Read the model definition and answer for the solid it produces. Units are mm, in the model's axes. Face numbers are marked on the shaded views. A direction names the side the tool comes from. Coordinates: 2 decimals unless noted, no trailing zeros. Write each loop counter-clockwise with the first axis right and the second up, starting at its lowest first coordinate (ties: lowest second). Pieces come first, ordered by that corner, then holes.
(1) Find the intervals of material crossed by probe 1 along Y at (x, z) = (38, -181.5); probe 2 along Z at (x, y) = (21, -173); probe 3 along X at (y, z) = (-77, -86.5), in increasing order.
(2) Which of the six approach directions +Z, -Z, +X, -X, +Y, -Y give full straight-line access (tool end or side, diameter ignored) to the marked faces 1 and 2?
(3) Section A-A on x = 16 is taken. Write down the section's boundary in (y, z).
(4) Section C-C on y = -151 is taken. Write down the section's boundary in (x, z).
(5) The mould has two halves that part along Z. Classify the marked faces 3, 4 and 5: +Z half, -Z half, draft (parallel to the pull), parting line (faces both ways), or undercut.
(6) Section B-B on z = -127.5 is taken. Write down the section's boundary in (x, y).
Autodesk Inventor part; units mm, degrees
ref_plane "YZ Plane" through (0, 0, 0) normal (1, 0, 0) x (0, 1, 0)
ref_plane "XZ Plane" through (0, 0, 0) normal (0, 1, 0) x (-1, 0, 0)
ref_plane "XY Plane" through (0, 0, 0) normal (0, 0, 1) x (1, 0, 0)
ref_plane "РабПлоскость1" through (8, 0, 0) normal (1, 0, 0) x (0, 0, -1)
sketch "Эскиз2" plane through (8, 0, 0) normal (1, 0, 0) x (0, 0, -1)
  line L0 (200, 300) -> (-200, 300)
  line L1 (200, -300) -> (200, 300)
  line L2 (-200, 300) -> (200, 300)
  line L3 (200, 300) -> (200, -300)
  line L4 (200, -300) -> (-200, -300)
  line L5 (-200, -300) -> (-200, 300)
  line L6 (-196, 296) -> (196, 296)
  line L7 (196, 296) -> (196, -296)
  line L8 (196, -296) -> (-196, -296)
  line L9 (-196, -296) -> (-196, 296)
  point P0 (0, 0)
  dimension "d4" = 4
  dimension "d5" = 4
  dimension "d6" = 4
  dimension "d7" = 4
extrude "Выдавливание2" add sketch "Эскиз2" along normal blind 50
sketch "Эскиз3" plane through (8, 0, 0) normal (-1, 0, 0) x (0, 0, 1)
  line L0 (-200, -300) -> (-200, 300)
  line L1 (200, 300) -> (200, -300)
  line L2 (-200, 300) -> (200, 300)
  line L3 (200, 300) -> (200, -300)
  line L4 (200, -300) -> (-200, -300)
  line L5 (-200, -300) -> (-200, 300)
  point P0 (0, 0)
extrude "Выдавливание3" add sketch "Эскиз3" along normal blind 4
equation "\"d5\" = d4"
equation "\"d6\" = d4"
equation "\"d7\" = d4"
properties part number "Задняя стенка"
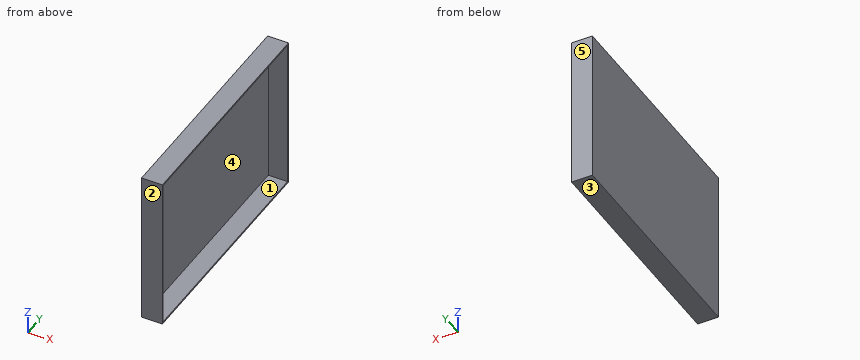
Response:
1. probe 1: y = -300 to -296, 296 to 300
1. probe 2: z = -200 to -196, 196 to 200
1. probe 3: x = 4 to 8
2. face 1: +X
2. face 2: +Z, -Z, +X, -X, -Y
3. outline: (-300, -200) - (300, -200) - (300, 200) - (-300, 200) - close; hole (-296, -196) - (296, -196) - (296, 196) - (-296, 196) - close
4. outline: (4, -200) - (58, -200) - (58, -196) - (8, -196) - (8, 196) - (58, 196) - (58, 200) - (4, 200) - close
5. face 3: -Z half
5. face 4: undercut
5. face 5: draft
6. outline: (4, -300) - (58, -300) - (58, -296) - (8, -296) - (8, 296) - (58, 296) - (58, 300) - (4, 300) - close
